from build123d import *

# Parameters (mm, degrees)
F1_DEPTH       = 12
F2_D           = 5
F2_DEPTH       = 15
F2_TIP         = 1.5021515476
F3_D           = 5
F3_DEPTH       = 15
F3_TIP         = 1.5021515476
F5_D           = 6.5
F5_DEPTH       = 10
F5_CBORE_D     = 8.2
F5_CBORE_DEPTH = 1
F5_TIP         = 1.9527970118
F6_D           = 3.2
F6_DEPTH       = 15
F6_TIP         = 0.9613769904
F7_D           = 3.2
F7_DEPTH       = 15
F7_TIP         = 0.9613769904


# Not quite as in the source:
# - a feature names something its author has since deleted; it is built from what else it names


with BuildPart() as f1:
    # F0 (on Top) → F1 (new body)
    with BuildSketch(Plane.XY):
        with BuildLine():
            Line((-19, -1.8754155822), (-19, 1.1245844178))
            Line((-19, 1.1245844178), (-15.8377223398, 1.1245844178))
            ThreePointArc((-15.8377223398, 1.1245844178), (-22.5, -0.3754155822), (-15.8377223398, -1.8754155822))
            Line((-15.8377223398, -1.8754155822), (-19, -1.8754155822))
        make_face()
        with BuildLine():
            Line((-15.8377223398, 1.1245844178), (-19, 1.1245844178))
            Line((-19, 1.1245844178), (-19, -1.8754155822))
            Line((-19, -1.8754155822), (-15.8377223398, -1.8754155822))
            ThreePointArc((-15.8377223398, -1.8754155822), (-15.5854742781, -1.144189993), (-15.5, -0.3754155822))
            ThreePointArc((-15.5, -0.3754155822), (-15.5854742781, 0.3933588286), (-15.8377223398, 1.1245844178))
        make_face()
        with BuildLine():
            Line((15.8377223398, 1.1245844178), (-15.8377223398, 1.1245844178))
            ThreePointArc((-15.8377223398, 1.1245844178), (-15.5854742781, 0.3933588286), (-15.5, -0.3754155822))
            ThreePointArc((-15.5, -0.3754155822), (-15.5854742781, -1.144189993), (-15.8377223398, -1.8754155822))
            Line((-15.8377223398, -1.8754155822), (15.8377223398, -1.8754155822))
            ThreePointArc((15.8377223398, -1.8754155822), (15.5, -0.3754155822), (15.8377223398, 1.1245844178))
        make_face()
        with BuildLine():
            ThreePointArc((22.5, -0.3754155822), (19.7687744108, 3.0391101397), (15.8377223398, 1.1245844178))
            Line((15.8377223398, 1.1245844178), (19, 1.1245844178))
            Line((19, 1.1245844178), (19, -1.8754155822))
            Line((19, -1.8754155822), (15.8377223398, -1.8754155822))
            ThreePointArc((15.8377223398, -1.8754155822), (19.7687744108, -3.7899413041), (22.5, -0.3754155822))
        make_face()
        with BuildLine():
            Line((19, 1.1245844178), (15.8377223398, 1.1245844178))
            ThreePointArc((15.8377223398, 1.1245844178), (15.5, -0.3754155822), (15.8377223398, -1.8754155822))
            Line((15.8377223398, -1.8754155822), (19, -1.8754155822))
            Line((19, -1.8754155822), (19, 1.1245844178))
        make_face()
    extrude(amount=F1_DEPTH)

    # F2
    with Locations(Plane(origin=(0, 0, 0), x_dir=(1, 0, 0), z_dir=(0, 0, -1))):
        with Locations((19, 0.3754155822)):
            Hole(F2_D / 2, depth=F2_DEPTH)
            with Locations((0, 0, -(F2_DEPTH + F2_TIP / 2))):  # 118° drill point
                Cone(0, F2_D / 2, F2_TIP, mode=Mode.SUBTRACT)

    # F3
    with Locations(Plane(origin=(0, 0, 0), x_dir=(1, 0, 0), z_dir=(0, 0, -1))):
        with Locations((-19, 0.3754155822)):
            Hole(F3_D / 2, depth=F3_DEPTH)
            with Locations((0, 0, -(F3_DEPTH + F3_TIP / 2))):  # 118° drill point
                Cone(0, F3_D / 2, F3_TIP, mode=Mode.SUBTRACT)

    # F5
    with Locations(Plane(origin=(0, 1.1245844178, 0), x_dir=(-1, 0, 0), z_dir=(0, 1, 0))):
        with Locations((0, 6)):
            CounterBoreHole(F5_D / 2, F5_CBORE_D / 2, F5_CBORE_DEPTH, depth=F5_DEPTH)
            with Locations((0, 0, -(F5_DEPTH + F5_TIP / 2))):  # 118° drill point
                Cone(0, F5_D / 2, F5_TIP, mode=Mode.SUBTRACT)

    # F6
    with Locations(Plane(origin=(0, 1.1245844178, 0), x_dir=(-1, 0, 0), z_dir=(0, 1, 0))):
        with Locations((-6, 6)):
            Hole(F6_D / 2, depth=F6_DEPTH)
            with Locations((0, 0, -(F6_DEPTH + F6_TIP / 2))):  # 118° drill point
                Cone(0, F6_D / 2, F6_TIP, mode=Mode.SUBTRACT)

    # F7
    with Locations(Plane(origin=(0, 1.1245844178, 0), x_dir=(-1, 0, 0), z_dir=(0, 1, 0))):
        with Locations((6, 6)):
            Hole(F7_D / 2, depth=F7_DEPTH)
            with Locations((0, 0, -(F7_DEPTH + F7_TIP / 2))):  # 118° drill point
                Cone(0, F7_D / 2, F7_TIP, mode=Mode.SUBTRACT)


solid = f1.part
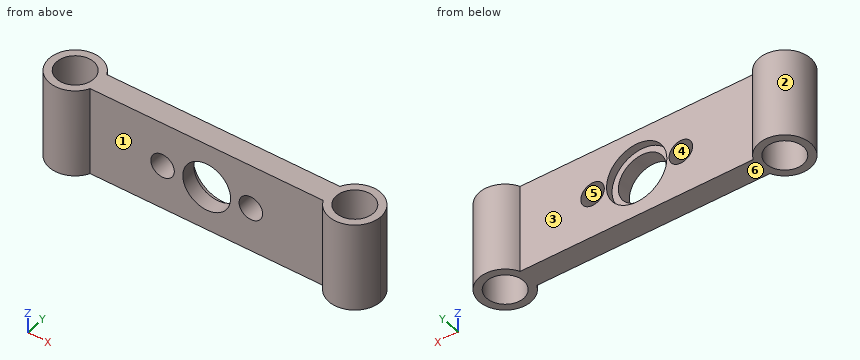
Geometry: final body of the model. Coordinates: model frame, mm. Face numbers are marked on the shaded views. A direction names the side the tool comes from. Give positions to 0.01 mm unless a question says otherwise; leave off trailing zeros. Write each loop counter-clockwise with the first axis right and the second up, starting at its lowest first coordinate (ties: lowest second). Pieces come first, ordered by that corner, then holes. Notation, with made-up numbers: M 26,35 L 35,35 A24 cw 35,64 Z; hole C 70.5,-38.5 d2. An arc over 180 degrees is marked long. Answer in a Markdown table with one row per item. Add a question column.
(1) Section C-C on z = 3.75. Return loops of the section in (x, y).
(2) Section A-A on z = 6. Return loops of the section in (x, y).
(3) First-contact query: pin 1 (4 mm diameter, centred on x = -6, z = 6, fed in from -Y); pin 2 (4 mm diameter, centred on x = 6, z = 6, fed in from +Y). Flat tips, straight axial feed; report the tip coordinate or a pass-through.
(4) Reachability of the marked faces 1, 2 and 3 from +Z, -Z, +X, -X, +Y, -Y: full face, straight path, thin tool, end or side. Return the list, or none.
(5) Mould query, pull axis X, two halves, no side actions, for the marked faces 4, 5 and 6. Classes: +X half, -X half, draft (parallel to the pull), parting line (faces both ways), or undercut.
(6) Section D-D on x = 0. Return loops of the section in (y, z), and give its area (3 significant figures).
(7) Ray query, line 1 (Y direction, x = -19, z = 7.25); line 2 (Z direction, x = 0, y = 0.6); line 3 (X direction, y = 0.5, z = 9.25). Return the intervals inside material, ascending.
(8) Section B-B on x = 19. Return loops of the section in (y, z).
Result set:
| question | item | result |
|---|---|---|
| 1 | outline | M -15.84,-1.88 L -2.35,-1.88 L -2.35,0.12 L -3.43,0.12 L -3.43,1.12 L -15.84,1.12 A3.5 ccw long Z; M 2.35,-1.88 L 15.84,-1.88 A3.5 ccw long 15.84,1.12 L 3.43,1.12 L 3.43,0.12 L 2.35,0.12 Z; hole C -19,-0.38 d5; hole C 19,-0.38 d5 |
| 2 | outline | M -15.84,-1.88 L -7.6,-1.88 L -7.6,1.12 L -15.84,1.12 A3.5 ccw long Z; M -4.4,-1.88 L -3.25,-1.88 L -3.25,0.12 L -4.1,0.12 L -4.1,1.12 L -4.4,1.12 Z; M 3.25,-1.88 L 4.4,-1.88 L 4.4,1.12 L 4.1,1.12 L 4.1,0.12 L 3.25,0.12 Z; M 7.6,-1.88 L 15.84,-1.88 A3.5 ccw long 15.84,1.12 L 7.6,1.12 Z; hole C -19,-0.38 d5; hole C 19,-0.38 d5 |
| 3 | pin 1 | stops at y = -1.88 |
| 3 | pin 2 | stops at y = 1.12 |
| 4 | face 1 | +Z, -Z, -Y |
| 4 | face 2 | +Z, -Z |
| 4 | face 3 | +Z, -Z, +Y |
| 5 | face 4 | undercut |
| 5 | face 5 | undercut |
| 5 | face 6 | draft |
| 6 | outline | M -1.88,0 L 1.12,0 L 1.12,1.9 L 0.12,1.9 L 0.12,2.75 L -1.88,2.75 Z; M -1.88,9.25 L 0.12,9.25 L 0.12,10.1 L 1.12,10.1 L 1.12,12 L -1.88,12 Z |
| 6 | area | 14.8 mm^2 |
| 7 | line 1 | y = -3.88 to -2.88, 2.12 to 3.12 |
| 7 | line 2 | z = 0 to 1.9, 10.1 to 12 |
| 7 | line 3 | x = -22.39 to -21.34, -16.66 to -2.5, 2.5 to 16.66, 21.34 to 22.39 |
| 8 | outline | M -3.88,0 L -2.88,0 L -2.88,12 L -3.88,12 Z; M 2.12,0 L 3.12,0 L 3.12,12 L 2.12,12 Z |
